from build123d import *

# Parameters (mm, degrees)
BOX035_W     = 9
BOX035_H     = 13
BOX035_DEPTH = 60
BOX023_W     = 9
BOX023_H     = 13
BOX023_DEPTH = 60
BOX024_W     = 9
BOX024_H     = 13
BOX024_DEPTH = 60
BOX025_W     = 9
BOX025_H     = 13
BOX025_DEPTH = 60
BOX026_W     = 9
BOX026_H     = 13
BOX026_DEPTH = 60
BOX027_W     = 9
BOX027_H     = 13
BOX027_DEPTH = 60
BOX028_W     = 9
BOX028_H     = 13
BOX028_DEPTH = 60
BOX029_W     = 9
BOX029_H     = 13
BOX029_DEPTH = 60
BOX030_W     = 9
BOX030_H     = 13
BOX030_DEPTH = 60
BOX031_W     = 9
BOX031_H     = 13
BOX031_DEPTH = 60
BOX032_W     = 9
BOX032_H     = 13
BOX032_DEPTH = 60
BOX033_W     = 9
BOX033_H     = 13
BOX033_DEPTH = 60
BOX034_W     = 9
BOX034_H     = 13
BOX034_DEPTH = 60
BOX036_W     = 9
BOX036_H     = 13
BOX036_DEPTH = 60
BOX037_W     = 9
BOX037_H     = 13
BOX037_DEPTH = 60
BOX038_W     = 9
BOX038_H     = 13
BOX038_DEPTH = 60
BOX039_W     = 9
BOX039_H     = 13
BOX039_DEPTH = 60
BOX022_W     = 9
BOX022_H     = 13
BOX022_DEPTH = 60
BOX021_W     = 200
BOX021_H     = 15
BOX021_DEPTH = 60


with BuildPart() as cube035:
    # Box035 → Box035 (new body)
    with BuildSketch(Plane(origin=(145, -15, 0), x_dir=(1, 0, 0), z_dir=(0, 0, 1))):
        with Locations((4.5, 6.5)):
            Rectangle(BOX035_W, BOX035_H)
    extrude(amount=BOX035_DEPTH)


with BuildPart() as cube023:
    # Box023 → Box023 (new body)
    with BuildSketch(Plane(origin=(13, -15, 0), x_dir=(1, 0, 0), z_dir=(0, 0, 1))):
        with Locations((4.5, 6.5)):
            Rectangle(BOX023_W, BOX023_H)
    extrude(amount=BOX023_DEPTH)


with BuildPart() as cube024:
    # Box024 → Box024 (new body)
    with BuildSketch(Plane(origin=(24, -15, 0), x_dir=(1, 0, 0), z_dir=(0, 0, 1))):
        with Locations((4.5, 6.5)):
            Rectangle(BOX024_W, BOX024_H)
    extrude(amount=BOX024_DEPTH)


with BuildPart() as cube025:
    # Box025 → Box025 (new body)
    with BuildSketch(Plane(origin=(35, -15, 0), x_dir=(1, 0, 0), z_dir=(0, 0, 1))):
        with Locations((4.5, 6.5)):
            Rectangle(BOX025_W, BOX025_H)
    extrude(amount=BOX025_DEPTH)


with BuildPart() as cube026:
    # Box026 → Box026 (new body)
    with BuildSketch(Plane(origin=(46, -15, 0), x_dir=(1, 0, 0), z_dir=(0, 0, 1))):
        with Locations((4.5, 6.5)):
            Rectangle(BOX026_W, BOX026_H)
    extrude(amount=BOX026_DEPTH)


with BuildPart() as cube027:
    # Box027 → Box027 (new body)
    with BuildSketch(Plane(origin=(57, -15, 0), x_dir=(1, 0, 0), z_dir=(0, 0, 1))):
        with Locations((4.5, 6.5)):
            Rectangle(BOX027_W, BOX027_H)
    extrude(amount=BOX027_DEPTH)


with BuildPart() as cube028:
    # Box028 → Box028 (new body)
    with BuildSketch(Plane(origin=(68, -15, 0), x_dir=(1, 0, 0), z_dir=(0, 0, 1))):
        with Locations((4.5, 6.5)):
            Rectangle(BOX028_W, BOX028_H)
    extrude(amount=BOX028_DEPTH)


with BuildPart() as cube029:
    # Box029 → Box029 (new body)
    with BuildSketch(Plane(origin=(79, -15, 0), x_dir=(1, 0, 0), z_dir=(0, 0, 1))):
        with Locations((4.5, 6.5)):
            Rectangle(BOX029_W, BOX029_H)
    extrude(amount=BOX029_DEPTH)


with BuildPart() as cube030:
    # Box030 → Box030 (new body)
    with BuildSketch(Plane(origin=(90, -15, 0), x_dir=(1, 0, 0), z_dir=(0, 0, 1))):
        with Locations((4.5, 6.5)):
            Rectangle(BOX030_W, BOX030_H)
    extrude(amount=BOX030_DEPTH)


with BuildPart() as cube031:
    # Box031 → Box031 (new body)
    with BuildSketch(Plane(origin=(101, -15, 0), x_dir=(1, 0, 0), z_dir=(0, 0, 1))):
        with Locations((4.5, 6.5)):
            Rectangle(BOX031_W, BOX031_H)
    extrude(amount=BOX031_DEPTH)


with BuildPart() as cube032:
    # Box032 → Box032 (new body)
    with BuildSketch(Plane(origin=(112, -15, 0), x_dir=(1, 0, 0), z_dir=(0, 0, 1))):
        with Locations((4.5, 6.5)):
            Rectangle(BOX032_W, BOX032_H)
    extrude(amount=BOX032_DEPTH)


with BuildPart() as cube033:
    # Box033 → Box033 (new body)
    with BuildSketch(Plane(origin=(123, -15, 0), x_dir=(1, 0, 0), z_dir=(0, 0, 1))):
        with Locations((4.5, 6.5)):
            Rectangle(BOX033_W, BOX033_H)
    extrude(amount=BOX033_DEPTH)


with BuildPart() as cube034:
    # Box034 → Box034 (new body)
    with BuildSketch(Plane(origin=(134, -15, 0), x_dir=(1, 0, 0), z_dir=(0, 0, 1))):
        with Locations((4.5, 6.5)):
            Rectangle(BOX034_W, BOX034_H)
    extrude(amount=BOX034_DEPTH)


with BuildPart() as cube036:
    # Box036 → Box036 (new body)
    with BuildSketch(Plane(origin=(156, -15, 0), x_dir=(1, 0, 0), z_dir=(0, 0, 1))):
        with Locations((4.5, 6.5)):
            Rectangle(BOX036_W, BOX036_H)
    extrude(amount=BOX036_DEPTH)


with BuildPart() as cube037:
    # Box037 → Box037 (new body)
    with BuildSketch(Plane(origin=(167, -15, 0), x_dir=(1, 0, 0), z_dir=(0, 0, 1))):
        with Locations((4.5, 6.5)):
            Rectangle(BOX037_W, BOX037_H)
    extrude(amount=BOX037_DEPTH)


with BuildPart() as cube038:
    # Box038 → Box038 (new body)
    with BuildSketch(Plane(origin=(178, -15, 0), x_dir=(1, 0, 0), z_dir=(0, 0, 1))):
        with Locations((4.5, 6.5)):
            Rectangle(BOX038_W, BOX038_H)
    extrude(amount=BOX038_DEPTH)


with BuildPart() as cube039:
    # Box039 → Box039 (new body)
    with BuildSketch(Plane(origin=(189, -15, 0), x_dir=(1, 0, 0), z_dir=(0, 0, 1))):
        with Locations((4.5, 6.5)):
            Rectangle(BOX039_W, BOX039_H)
    extrude(amount=BOX039_DEPTH)


with BuildPart() as compound001:
    # Box022 → Box022 (new body)
    with BuildSketch(Plane(origin=(2, -15, 0), x_dir=(1, 0, 0), z_dir=(0, 0, 1))):
        with Locations((4.5, 6.5)):
            Rectangle(BOX022_W, BOX022_H)
    extrude(amount=BOX022_DEPTH)

    # Compound001: union Cube035, Cube023, Cube024, Cube025, Cube026, Cube027, Cube028, Cube029, Cube030, Cube031, Cube032, Cube033, Cube034, Cube036, Cube037, Cube038, Cube039
    add(cube035.part)
    add(cube023.part)
    add(cube024.part)
    add(cube025.part)
    add(cube026.part)
    add(cube027.part)
    add(cube028.part)
    add(cube029.part)
    add(cube030.part)
    add(cube031.part)
    add(cube032.part)
    add(cube033.part)
    add(cube034.part)
    add(cube036.part)
    add(cube037.part)
    add(cube038.part)
    add(cube039.part)


with BuildPart() as cut002:
    # Box021 → Box021 (new body)
    with BuildSketch(Plane(origin=(0, -15, 0), x_dir=(1, 0, 0), z_dir=(0, 0, 1))):
        with Locations((100, 7.5)):
            Rectangle(BOX021_W, BOX021_H)
    extrude(amount=BOX021_DEPTH)

    # Cut002: cut Compound001
    add(compound001.part, mode=Mode.SUBTRACT)


solid = cut002.part
Can you work these out from the model? Positions are in its coordinate system, mm. Round coordinates to 2 decimals unless told otherwise and drop trailing zeros. Write each loop counter-clockwise with the first axis right and the second up, starting at its lowest first coordinate (ties: lowest second). Pieces come first, ordered by that corner, then holes. Notation, with made-up numbers: M 80.25,84.5 L 128.25,84.5 A28 ccw 128.25,115.5 Z; hole C -23.5,-21.5 d11. An arc over 180 degrees is marked long. Use a Markdown table: item, result.
Item 1: For pin 1 Ø4.5 at (x, z) = (72, 19) entering from -Y, with a flat end and sliding along its axis, tell me the tip position at first contact or that it passes through.
Found:
| item | result |
|---|---|
| pin 1 | stops at y = -2 |
Item 2: If I drill on line 1 along Y through (x, z) = (75.5, 33), over which ranges is the centre line in solid material (lowest first)? Write a range as [from, to].
Found:
| item | result |
|---|---|
| line 1 | y = [-2, 0] |
Item 3: I want a section at B-B (y = -10.25). State how many separate pieces and enclosed holes the cut face has, and give its area (3 significant figures).
Found:
| item | result |
|---|---|
| separate pieces | 19 |
| enclosed holes | 0 |
| area | 2,280 mm2 |
Item 4: I want a section at A-A (x = 139). List the corners of the cut face in (y, z) for me, and give its area (3 significant figures).
Found:
| item | result |
|---|---|
| outline | M -2,0 L 0,0 L 0,60 L -2,60 Z |
| area | 120 mm2 |
